Work out the finished part from the listing and answer in its coordinate system (mm). Coordinates: 2 decimals unless noted, no trailing zeros. Order: outer loops, then holes, each group sorted by start corner. A loop starts at its lowest first (then second) coordinate and runs counter-clockwise, first axis right, second up. Notation, with made-up numbers: M 67,-32.75 L 82,-32.75 A19 cw 82,-5.75 Z; hole C 39.5,60 d9. An arc over 180 degrees is marked long. Use a Markdown table: item, result.
from build123d import *

# Parameters (mm, degrees)
SKETCH1_W           = 140
SKETCH1_H           = 90
SKETCH1_R           = 2
SKETCH1_R_2         = 13.5
BOSS_EXTRUDE1_DEPTH = 4
SKETCH2_R           = 2
CUT_EXTRUDE1_DEPTH  = 5
SKETCH3_R           = 2
CUT_EXTRUDE2_DEPTH  = 5


with BuildPart() as part:
    # Sketch1 → Boss-Extrude1 (new body)
    with BuildSketch(Plane.XY):
        Rectangle(SKETCH1_W, SKETCH1_H)
        with Locations((0, -2.5)):
            Circle(SKETCH1_R, mode=Mode.SUBTRACT)
        with Locations((17.5, -20)):
            Circle(SKETCH1_R, mode=Mode.SUBTRACT)
        with Locations((0, -37.5)):
            Circle(SKETCH1_R, mode=Mode.SUBTRACT)
        with Locations((-17.5, -20)):
            Circle(SKETCH1_R, mode=Mode.SUBTRACT)
        with Locations((0, -20)):
            Circle(SKETCH1_R_2, mode=Mode.SUBTRACT)
    extrude(amount=BOSS_EXTRUDE1_DEPTH)

    # Sketch2 → Cut-Extrude1 (cut, through all)
    with BuildSketch(Plane.XY.offset(4)):
        with Locations((0, 35)):
            Circle(SKETCH2_R)
        with Locations((-60, 35)):
            Circle(SKETCH2_R)
        with Locations((60, 35)):
            Circle(SKETCH2_R)
    extrude(amount=-CUT_EXTRUDE1_DEPTH, mode=Mode.SUBTRACT)

    # Sketch3 → Cut-Extrude2 (cut, through all)
    with BuildSketch(Plane.XY.offset(4)):
        with Locations((-60, -25)):
            Circle(SKETCH3_R)
        with Locations((-60, -85)):
            Circle(SKETCH3_R)
        with Locations((60, -85)):
            Circle(SKETCH3_R)
        with Locations((60, -25)):
            Circle(SKETCH3_R)
    extrude(amount=-CUT_EXTRUDE2_DEPTH, mode=Mode.SUBTRACT)


solid = part.part
(1) A cutting plane is placed at A-A (y = -20). Determine the outline of the cut face in (x, z), then the cut area to 3 significant figures.
Conclusion:
| item | result |
|---|---|
| outline | M -70,0 L -19.5,0 L -19.5,4 L -70,4 Z; M -15.5,0 L -13.5,0 L -13.5,4 L -15.5,4 Z; M 13.5,0 L 15.5,0 L 15.5,4 L 13.5,4 Z; M 19.5,0 L 70,0 L 70,4 L 19.5,4 Z |
| area | 420 mm2 |
(2) Straight lines are drawn through the part: L1, parallel to Y at x = 60, z = 0.85; L2, parallel to Y at x = 0, z = 2.2; L3, parallel to X at y = -21, z = 2.65. For each, find the intervals that lie inside material, in ascending order.
Conclusion:
| item | result |
|---|---|
| L1 | -45 to -27, -23 to 33, 37 to 45 |
| L2 | -45 to -39.5, -35.5 to -33.5, -6.5 to -4.5, -0.5 to 33, 37 to 45 |
| L3 | -70 to -19.23, -15.77 to -13.46, 13.46 to 15.77, 19.23 to 70 |
(3) A cutting plane is placed at B-B (x = -60). Determine the outline of the cut face in (y, z), then the cut area to 3 significant figures.
Conclusion:
| item | result |
|---|---|
| outline | M -45,0 L -27,0 L -27,4 L -45,4 Z; M -23,0 L 33,0 L 33,4 L -23,4 Z; M 37,0 L 45,0 L 45,4 L 37,4 Z |
| area | 328 mm2 |
(4) A cutting plane is placed at D-D (y = -11). Determine the outline of the cut face in (x, z).
Conclusion:
| item | result |
|---|---|
| outline | M -70,0 L -10.06,0 L -10.06,4 L -70,4 Z; M 10.06,0 L 70,0 L 70,4 L 10.06,4 Z |
(5) A cutting plane is placed at C-C (z = 1.35). Give the number of separate pieces and of enclosed holes in the cut face, then the cut area to 3 significant figures.
Conclusion:
| item | result |
|---|---|
| separate pieces | 1 |
| enclosed holes | 10 |
| area | 11,900 mm2 |
(6) Determine the mould class of faces 1 (the cylindrical face through (0, 33, 2)), 2 (the flat face through (-70, -1, 2)), 3 (the flat face through (-1, 45, 2)) for opening direction X: pulls with the +X half, pulls with the -X half, needs draft (parallel to the pull), parting line crosses it, or undercut.
Conclusion:
| item | result |
|---|---|
| face 1 | undercut |
| face 2 | pulls with the -X half |
| face 3 | needs draft |
